Geometry: final body of the model. Coordinates: model frame, mm. Face numbers are marked on the shaded views. A direction names the side the tool comes from. Give positions to 0.01 mm unless a question says otherwise; leave off trailing zeros. Loops run counter-clockwise (first coordinate to the right, second up) from the corner with the lowest first, then second, coordinate; pieces in that order, holes last. Notation, with made-up numbers: (81.5, 85.5) -> (102.5, 85.5) arc R22 cw to (102.5, 112.5) -> close; hole circle Ø1 at (41.25, -21). An arc over 180 degrees is marked (long way). Answer in a Markdown table with one row per item. Add a question column.
from build123d import *

# Parameters (mm, degrees)
BOSS_EXTRUDE1_DEPTH = 1.5
SKETCH2_OUTSIDE_W   = 18.614
SKETCH2_OUTSIDE_H   = 18.614
SKETCH2_OUTSIDE_R   = 2.075826116
CUT_EXTRUDE1_DEPTH  = 3
CUT_EXTRUDE1_TAPER  = 60
SKETCH3_R           = 2.375
BOSS_EXTRUDE2_DEPTH = 2
CUT_EXTRUDE3_START  = -1
SKETCH5_OUTSIDE_W   = 8.424
SKETCH5_OUTSIDE_H   = 8.424
SKETCH5_OUTSIDE_R   = 2.075826116
CUT_EXTRUDE3_DEPTH  = 1
CHAMFER1_SIZE       = 0.1
SKETCH6_R           = 1
CUT_EXTRUDE4_DEPTH  = 4
CHAMFER2_SIZE       = 0.3


with BuildPart() as part:
    # Sketch1 → Boss-Extrude1 (new body, symmetric)
    with BuildSketch(Plane.XY):
        Polygon((-0.324730748, 2.050269252), (0, 2.375), (0.324730748, 2.050269252), (0.733915362, 2.258759226), (0.942405336, 1.849574613), (1.395989974, 1.921415362), (1.467830723, 1.467830723), (1.921415362, 1.395989974), (1.849574613, 0.942405336), (2.258759226, 0.733915362), (2.050269252, 0.324730748), (2.375, 0), (2.050269252, -0.324730748), (2.258759226, -0.733915362), (1.849574613, -0.942405336), (1.921415362, -1.395989974), (1.467830723, -1.467830723), (1.395989974, -1.921415362), (0.942405336, -1.849574613), (0.733915362, -2.258759226), (0.324730748, -2.050269252), (0, -2.375), (-0.324730748, -2.050269252), (-0.733915362, -2.258759226), (-0.942405336, -1.849574613), (-1.395989974, -1.921415362), (-1.467830723, -1.467830723), (-1.921415362, -1.395989974), (-1.849574613, -0.942405336), (-2.258759226, -0.733915362), (-2.050269252, -0.324730748), (-2.375, 0), (-2.050269252, 0.324730748), (-2.258759226, 0.733915362), (-1.849574613, 0.942405336), (-1.921415362, 1.395989974), (-1.467830723, 1.467830723), (-1.395989974, 1.921415362), (-0.942405336, 1.849574613), (-0.733915362, 2.258759226), align=None)
    extrude(amount=BOSS_EXTRUDE1_DEPTH, both=True)

    # Sketch2 outside → Cut-Extrude1 (cut)
    with BuildSketch(Plane.XY.offset(1.5)):
        Rectangle(SKETCH2_OUTSIDE_W, SKETCH2_OUTSIDE_H)
        Circle(SKETCH2_OUTSIDE_R, mode=Mode.SUBTRACT)
    cut_extrude1 = extrude(amount=-CUT_EXTRUDE1_DEPTH, taper=CUT_EXTRUDE1_TAPER, mode=Mode.SUBTRACT)

    # Mirror1: Cut-Extrude1 across plane
    add(cut_extrude1.mirror(Plane.XY), mode=Mode.SUBTRACT)

    # Sketch3 → Boss-Extrude2 (add)
    with BuildSketch(Plane(origin=(0, 0, -1.5), x_dir=(-1, 0, 0), z_dir=(0, 0, -1))):
        Circle(SKETCH3_R)
    extrude(amount=BOSS_EXTRUDE2_DEPTH)

    # Sketch5 outside → Cut-Extrude3 (cut)
    with BuildSketch(Plane(origin=(0, 0, -3.5), x_dir=(-1, 0, 0), z_dir=(0, 0, -1)).offset(CUT_EXTRUDE3_START)):
        Rectangle(SKETCH5_OUTSIDE_W, SKETCH5_OUTSIDE_H)
        Circle(SKETCH5_OUTSIDE_R, mode=Mode.SUBTRACT)
    extrude(amount=-CUT_EXTRUDE3_DEPTH, mode=Mode.SUBTRACT)

    # Chamfer1
    chamfer1_edges = [part.edges().sort_by_distance(p)[0] for p in [
        (2.375, 0, -2.5),
    ]]
    chamfer(chamfer1_edges, length=CHAMFER1_SIZE)

    # Sketch6 → Cut-Extrude4 (cut)
    with BuildSketch(Plane.XY.offset(1.5)):
        Circle(SKETCH6_R)
    extrude(amount=-CUT_EXTRUDE4_DEPTH, mode=Mode.SUBTRACT)

    # Chamfer2
    chamfer2_edges = [part.edges().sort_by_distance(p)[0] for p in [
        (-1, 0, 1.5),
    ]]
    chamfer(chamfer2_edges, length=CHAMFER2_SIZE)


solid = part.part
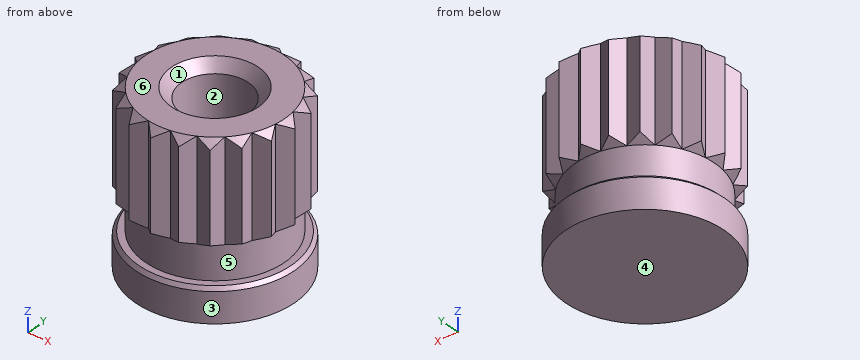
(1) Pin query (flat end, axial travel): pin 1 Ø1.6 at (x, y) = (0, 0) entering from +Z; pin 2 Ø1.5 at (x, z) = (-1, -0.5) entering from +Y; pin 3 Ø2 at (x, z) = (1, -2) entering from -Y. Return the tip coordinate at first contact, or that it passes through.
(2) Cut plane A-A on z = -2. Return the cut outline in (x, y), then the cut area to 3 significant figures.
(3) Draft query along X for the marked faces 1, 2, 3 and 4. Return one class per face: +X half, -X half, draft (parallel to the pull), parting line (faces both ways), or undercut.
(4) Material intervals for line 1 along Y through (x, z) = (0, -1.65); line 2 along Z through (x, y) = (0.7, 0.6); line 3 along X through (y, z) = (0.4, 0.95), sorted ascending. Write a range as from..to.
(5) Reachability of the marked faces 5 and 6 from +Z, -Z, +X, -X, +Y, -Y: full face, straight path, thin tool, end or side. Return the list, or none.
Answer list:
| question | item | result |
|---|---|---|
| 1 | pin 1 | stops at z = -2.5 |
| 1 | pin 2 | stops at y = 2.26 |
| 1 | pin 3 | stops at y = -2.37 |
| 2 | outline | circle Ø4.15 at (0, 0); hole circle Ø2 at (0, 0) |
| 2 | area | 10.4 mm² |
| 3 | face 1 | undercut |
| 3 | face 2 | undercut |
| 3 | face 3 | parting line |
| 3 | face 4 | draft |
| 4 | line 1 | y = -2.08..-1, 1..2.08 |
| 4 | line 2 | z = -3.5..-2.5 |
| 4 | line 3 | x = -2.09..-0.92, 0.92..2.09 |
| 5 | face 5 | none |
| 5 | face 6 | +Z, +X, -X, +Y, -Y |
